Could you check a few things on this model? Use its own coordinates, in mm. A direction names the side the tool comes from. Give positions to 0.01 mm unless a question says otherwise; leave off trailing zeros. Order: outer loops, then holes, each group sorted by start corner. A loop starts at its lowest first (then second) coordinate and runs counter-clockwise, first axis right, second up. Notation, with made-up numbers: M 67,32.5 L 95,32.5 A21 ccw 95,49.5 Z; hole C 19.5,31.25 d6. An arc over 180 degrees is marked long. Use a Markdown table: item, result. Add a question column.
Autodesk Inventor part; units mm, degrees
ref_plane "YZ Plane" through (0, 0, 0) normal (1, 0, 0) x (0, 1, 0)
ref_plane "XZ Plane" through (0, 0, 0) normal (0, 1, 0) x (-1, 0, 0)
ref_plane "XY Plane" through (0, 0, 0) normal (0, 0, 1) x (1, 0, 0)
sketch "Sketch1" plane through (0, 0, 0) normal (0, 0, 1) x (1, 0, 0)
  line L0 (0.039, 0.2446) -> (0.039, 3.6446)
  line L1 (-3.961, 12.0746) -> (-3.961, 0.2446)
  line L2 (-3.961, 0.2446) -> (0.039, 0.2446)
  line L3 (6.039, 3.6446) -> (30.489, 3.6446)
  line L4 (-3.961, 12.0746) -> (-0.45, 12.0746)
  line L5 (-0.45, 12.0746) -> (-0.45, 8.6446)
  line L6 (0.039, 3.6446) -> (6.039, 3.6446)
  line L7 (-0.45, 8.6446) -> (37.489, 8.6446)
  line L8 (30.489, 3.6446) -> (30.489, -1.7694)
  line L9 (37.489, -1.7694) -> (37.489, 8.6446)
  line L10 (30.489, -1.7694) -> (32, -1.7694)
  line L11 (32, -1.7694) -> (32, -7.6694)
  line L12 (32, -7.6694) -> (35, -7.6694)
  line L13 (35, -7.6694) -> (35, -1.7694)
  line L14 (35, -1.7694) -> (37.489, -1.7694)
  dimension "d0" = 6
  dimension "d10" = 4
  dimension "d22" = 3.4
  dimension "d23" = 3.43
  dimension "d24" = 5
  dimension "d25" = 24.45
  dimension "d26" = 7
  dimension "d31" = 5.9
  dimension "d32" = 3
  dimension "d33" = 1.511
  dimension "d36" = 5.414
extrude "Extrusion1" add sketch "Sketch1" along normal blind 3
fillet "Fillet5" radius 2 1 edges at (37.489, 8.6446, 1.5)
fillet "Fillet6" radius 3 2 edges at (-3.961, 12.0746, 1.5) (-3.961, 0.2446, 1.5)
properties part number "Gripper V 8.0 servo bracket side left 3mm"
1) Please list where these lines run through material, in increasing order: line 1 (Y direction, x = 12.5, z = 0.4); line 2 (X direction, y = -4.5, z = 1.8); line 3 (X direction, y = 8.75, z = 1). Write a range as from..to.
2) Suppose I cut it at A-A on z = 2.4. Please give me the cut outline in (x, y), and give its area (3 significant figures).
3) Suppose I cut it at B-B on y = -2.5. Please give me the cut outline in (x, z).
4) Suppose I cut it at C-C on x = 16. Please give me the cut outline in (y, z).
5) For faces 1 (the face through (-0.45, 10, 1)), 2 (the face through (15, 3.645, 1)), 3 (the face through (35, -5, 1)), which set-ups out of +Z, -Z, +X, -X, +Y, -Y let a thin tool reach every point of the face, with its end or its side?
6) We'd pull the mould along X, two halves only. Please class faces 4 (the face through (-0.5, 0.245, 1.5)), 5 (the face through (-3.11, 1.15, 1.52)), 6 (the face through (30.489, 1, 1)): pulls with the +X half, pulls with the -X half, needs draft (parallel to the pull), parting line crosses it, or undercut.
7) For pin 1 (1.5 mm diameter, centred on x = 15, z = 2, fed in from -Y); pin 2 (1.2 mm diameter, centred on x = 36.5, z = 1.5, fed in from -Y); pin 3 (0.9 mm diameter, centred on y = -3.5, z = 1, fed in from +X), each with a flat end and sliding along its axis, tell me the tip position at first contact or that it passes through.
Values found:
| question | item | result |
|---|---|---|
| 1 | line 1 | y = 3.64..8.64 |
| 1 | line 2 | x = 32..35 |
| 1 | line 3 | x = -3.96..-0.45 |
| 2 | outline | M -3.96,3.24 A3 ccw -0.96,0.24 L 0.04,0.24 L 0.04,3.64 L 30.49,3.64 L 30.49,-1.77 L 32,-1.77 L 32,-7.67 L 35,-7.67 L 35,-1.77 L 37.49,-1.77 L 37.49,6.64 A2 ccw 35.49,8.64 L -0.45,8.64 L -0.45,12.07 L -0.96,12.07 A3 ccw -3.96,9.07 Z |
| 2 | area | 284 mm^2 |
| 3 | outline | M 32,0 L 35,0 L 35,3 L 32,3 Z |
| 4 | outline | M 3.64,0 L 8.64,0 L 8.64,3 L 3.64,3 Z |
| 5 | face 1 | +Z, -Z, +X, +Y |
| 5 | face 2 | +Z, -Z, -Y |
| 5 | face 3 | +Z, -Z, +X, -Y |
| 6 | face 4 | needs draft |
| 6 | face 5 | pulls with the -X half |
| 6 | face 6 | undercut |
| 7 | pin 1 | stops at y = 3.64 |
| 7 | pin 2 | stops at y = -1.77 |
| 7 | pin 3 | stops at x = 35 |
